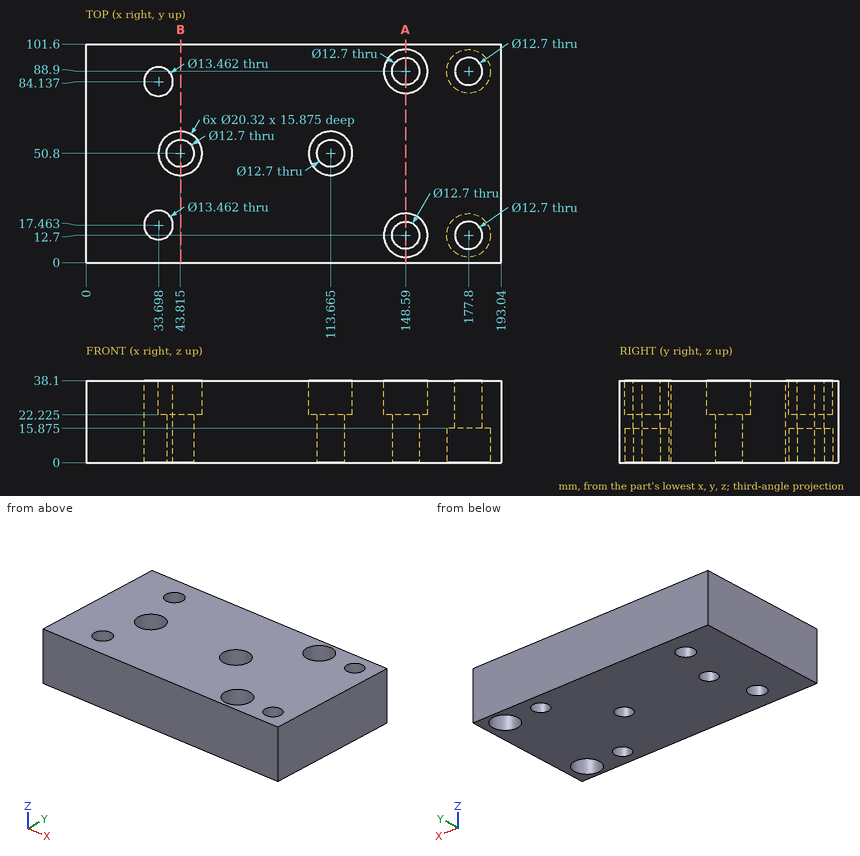
Part print with two shaded views. Sizes in mm from the minimum x, y, z corner. Round coordinates to 2 decimals unless told otherwise and drop trailing zeros. Loops run counter-clockwise (first coordinate to the right, second up) from the corner with the lowest first, then second, coordinate; pieces in that order, holes last. Notation, with made-up numbers: (52.25, 84) - (97.25, 84) arc R11 ccw to (97.25, 93) - close; hole circle Ø9 at (18, -31). An arc over 180 degrees is marked (long way). Answer as a JSON object with one key per item and string values.
Item 1: Wall check: L1, parallel to Y at x = 148, z = 15; L2, parallel to Y at x = 177.8, z = 7; L3, parallel to X at y = 12, z = 9 (1 decimal). Give the ranges that are in metal, low to high.
Output:
{"L1": "0 to 6.38, 19.02 to 82.58, 95.22 to 101.6", "L2": "0 to 2.54, 22.86 to 78.74, 99.06 to 101.6", "L3": "0 to 29.8, 37.6 to 142.3, 154.9 to 167.7, 187.9 to 193"}
Item 2: Band-saw the part on A-A on x = 148.59. State how many separate pieces and enclosed holes the cut face has, plus the area to 3 significant figures.
Output:
{"separate pieces": "3", "enclosed holes": "0", "area": "2,660 mm2"}
Item 3: Band-saw the part on B-B on x = 44. List the corners of the cut face in (y, z) (1 decimal), plus the area to 3 significant figures.
Output:
{"outline": "(0, 0) - (44.5, 0) - (44.5, 22.2) - (40.6, 22.2) - (40.6, 38.1) - (0, 38.1) - close; (57.1, 0) - (101.6, 0) - (101.6, 38.1) - (61, 38.1) - (61, 22.2) - (57.1, 22.2) - close", "area": "3,270 mm2"}
Item 4: Pin check, flat tips, straight feed: pin 1 (16.5 mm diameter, centred on x = 148.59, y = 88.9, fed in from +Z) (1 decimal); pin 2 (10 mm diameter, centred on x = 148.59, y = 12.7, fed in from +Z); pin 3 (6 mm diameter, centred on x = 181.5, y = 12.5, fed in from -Z) (1 decimal). Stop position of each tip, or through.
Output:
{"pin 1": "z = 22.2", "pin 2": "through", "pin 3": "z = 15.9"}
